Input: part model. Units: mm. Frame: model coordinates. Face numbers are marked on the shaded views. Round coordinates to 2 decimals unless told otherwise and drop trailing zeros. Loops run counter-clockwise (first coordinate to the right, second up) from the corner with the lowest first, then second, coordinate; pieces in that order, holes last. Notation, with made-up numbers: (86.5, -21) - (91.5, -21) arc R29 ccw to (91.5, 17) - close; hole circle Ø8 at (-18, 19). An arc over 180 degrees is marked (long way). One line per question, with ' | ' between items. Start each with the question number.
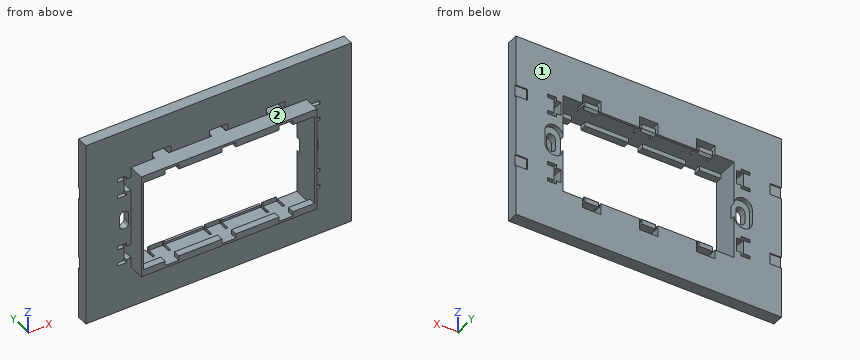
from build123d import *

# Parameters (mm, degrees)
CROQUIS1_W              = 116.45
CROQUIS1_H              = 82
SALIENTE_EXTRUIR2_DEPTH = 5
CROQUIS2_W              = 74.95
CROQUIS2_H              = 44
CORTAR_EXTRUIR1_DEPTH   = 5
CROQUIS3_W              = 76.95
CROQUIS3_H              = 46
CROQUIS3_W_2            = 74.95
CROQUIS3_H_2            = 44
SALIENTE_EXTRUIR3_DEPTH = 7
CROQUIS4_W              = 74.95
CROQUIS4_H              = 3
SALIENTE_EXTRUIR4_DEPTH = 3
CROQUIS5_W              = 3
CROQUIS5_H              = 2
CORTAR_EXTRUIR9_DEPTH   = 3
CROQUIS9_W              = 6
CROQUIS9_H              = 3
CORTAR_EXTRUIR10_DEPTH  = 1
CROQUIS10_W             = 74.95
CROQUIS10_H             = 3
CORTAR_EXTRUIR11_DEPTH  = 1
CROQUIS11_W             = 6
CROQUIS11_H             = 3
CORTAR_EXTRUIR12_DEPTH  = 1
CROQUIS12_W             = 74.95
CROQUIS12_H             = 3
CORTAR_EXTRUIR13_DEPTH  = 1
CROQUIS13_W             = 1
CROQUIS13_H             = 5
CORTAR_EXTRUIR21_DEPTH  = 4
CROQUIS14_W             = 1
CROQUIS14_H             = 5
CORTAR_EXTRUIR22_DEPTH  = 4
CROQUIS15_W             = 8
CROQUIS15_H             = 3
CORTAR_EXTRUIR23_DEPTH  = 16
SALIENTE_EXTRUIR8_DEPTH = 70
SALIENTE_EXTRUIR9_DEPTH = 70
CROQUIS18_W             = 19
CROQUIS18_H             = 42
CORTAR_EXTRUIR24_DEPTH  = 8
CROQUIS19_W             = 9.475
CROQUIS19_H             = 44
CORTAR_EXTRUIR26_DEPTH  = 8
CROQUIS20_W             = 1
CROQUIS20_H             = 44
CORTAR_EXTRUIR27_DEPTH  = 4
CROQUIS21_W             = 5
CROQUIS21_H             = 5
CORTAR_EXTRUIR28_DEPTH  = 0.5
CORTAR_EXTRUIR29_DEPTH  = 5
CORTAR_EXTRUIR30_DEPTH  = 2
CORTAR_EXTRUIR31_DEPTH  = 5


with BuildPart() as part:
    # Croquis1 → Saliente-Extruir2 (new body)
    with BuildSketch(Plane(origin=(0, 0, 0), x_dir=(1, 0, 0), z_dir=(0, 1, 0))):
        Rectangle(CROQUIS1_W, CROQUIS1_H)
    extrude(amount=SALIENTE_EXTRUIR2_DEPTH)

    # Croquis2 → Cortar-Extruir1 (cut)
    with BuildSketch(Plane(origin=(0, 5, 0), x_dir=(1, 0, 0), z_dir=(0, 1, 0))):
        Rectangle(CROQUIS2_W, CROQUIS2_H)
    extrude(amount=-CORTAR_EXTRUIR1_DEPTH, mode=Mode.SUBTRACT)

    # Croquis3 → Saliente-Extruir3 (add)
    with BuildSketch(Plane.XZ):
        Rectangle(CROQUIS3_W, CROQUIS3_H)
        Rectangle(CROQUIS3_W_2, CROQUIS3_H_2, mode=Mode.SUBTRACT)
    extrude(amount=SALIENTE_EXTRUIR3_DEPTH)

    # Croquis4 → Saliente-Extruir4 (add)
    with BuildSketch(Plane.XZ.offset(7)):
        with Locations((0, 20.5)):
            Rectangle(CROQUIS4_W, CROQUIS4_H)
        with Locations((0, -20.5)):
            Rectangle(CROQUIS4_W, CROQUIS4_H)
    extrude(amount=-SALIENTE_EXTRUIR4_DEPTH)

    # Croquis5 → Cortar-Extruir9 (cut)
    with BuildSketch(Plane.XZ.offset(7)):
        Polygon((25, -19), (22, -19), (22, -21), (28, -21), (28, -19), align=None)
        Polygon((22, 21), (22, 19), (25, 19), (28, 19), (28, 21), align=None)
        with Locations((1.5, 20)):
            Rectangle(CROQUIS5_W, CROQUIS5_H)
        with Locations((-1.5, 20)):
            Rectangle(CROQUIS5_W, CROQUIS5_H)
        with Locations((-1.5, -20)):
            Rectangle(CROQUIS5_W, CROQUIS5_H)
        with Locations((1.5, -20)):
            Rectangle(CROQUIS5_W, CROQUIS5_H)
        Polygon((-22, -21), (-22, -19), (-25, -19), (-28, -19), (-28, -21), align=None)
        Polygon((-25, 19), (-22, 19), (-22, 21), (-28, 21), (-28, 19), align=None)
    extrude(amount=-CORTAR_EXTRUIR9_DEPTH, mode=Mode.SUBTRACT)

    # Croquis9 → Cortar-Extruir10 (cut)
    with BuildSketch(Plane(origin=(0, 0, 21), x_dir=(-1, 0, 0), z_dir=(0, 0, -1))):
        with Locations((25, -5.5)):
            Rectangle(CROQUIS9_W, CROQUIS9_H)
        with Locations((0, -5.5)):
            Rectangle(CROQUIS9_W, CROQUIS9_H)
        with Locations((-25, -5.5)):
            Rectangle(CROQUIS9_W, CROQUIS9_H)
    extrude(amount=-CORTAR_EXTRUIR10_DEPTH, mode=Mode.SUBTRACT)

    # Croquis10 → Cortar-Extruir11 (cut)
    with BuildSketch(Plane(origin=(0, 0, 19), x_dir=(-1, 0, 0), z_dir=(0, 0, -1))):
        with Locations((0, -5.5)):
            Rectangle(CROQUIS10_W, CROQUIS10_H)
    extrude(amount=-CORTAR_EXTRUIR11_DEPTH, mode=Mode.SUBTRACT)

    # Croquis11 → Cortar-Extruir12 (cut)
    with BuildSketch(Plane.XY.offset(-21)):
        with Locations((25, -5.5)):
            Rectangle(CROQUIS11_W, CROQUIS11_H)
        with Locations((0, -5.5)):
            Rectangle(CROQUIS11_W, CROQUIS11_H)
        with Locations((-25, -5.5)):
            Rectangle(CROQUIS11_W, CROQUIS11_H)
    extrude(amount=-CORTAR_EXTRUIR12_DEPTH, mode=Mode.SUBTRACT)

    # Croquis12 → Cortar-Extruir13 (cut)
    with BuildSketch(Plane.XY.offset(-19)):
        with Locations((0, -5.5)):
            Rectangle(CROQUIS12_W, CROQUIS12_H)
    extrude(amount=-CORTAR_EXTRUIR13_DEPTH, mode=Mode.SUBTRACT)

    # Croquis13 → Cortar-Extruir21 (cut)
    with BuildSketch(Plane.XY.offset(-22)):
        with Locations((21.5, 2.5)):
            Rectangle(CROQUIS13_W, CROQUIS13_H)
        with Locations((3.5, 2.5)):
            Rectangle(CROQUIS13_W, CROQUIS13_H)
        with Locations((-3.5, 2.5)):
            Rectangle(CROQUIS13_W, CROQUIS13_H)
        with Locations((-28.5, 2.5)):
            Rectangle(CROQUIS13_W, CROQUIS13_H)
        with Locations((-21.5, 2.5)):
            Rectangle(CROQUIS13_W, CROQUIS13_H)
        with Locations((28.5, 2.5)):
            Rectangle(CROQUIS13_W, CROQUIS13_H)
    extrude(amount=-CORTAR_EXTRUIR21_DEPTH, mode=Mode.SUBTRACT)

    # Croquis14 → Cortar-Extruir22 (cut)
    with BuildSketch(Plane(origin=(0, 0, 22), x_dir=(-1, 0, 0), z_dir=(0, 0, -1))):
        with Locations((28.5, 2.5)):
            Rectangle(CROQUIS14_W, CROQUIS14_H)
        with Locations((-21.5, 2.5)):
            Rectangle(CROQUIS14_W, CROQUIS14_H)
        with Locations((21.5, 2.5)):
            Rectangle(CROQUIS14_W, CROQUIS14_H)
        with Locations((3.5, 2.5)):
            Rectangle(CROQUIS14_W, CROQUIS14_H)
        with Locations((-3.5, 2.5)):
            Rectangle(CROQUIS14_W, CROQUIS14_H)
        with Locations((-28.5, 2.5)):
            Rectangle(CROQUIS14_W, CROQUIS14_H)
    extrude(amount=-CORTAR_EXTRUIR22_DEPTH, mode=Mode.SUBTRACT)

    # Croquis15 → Cortar-Extruir23 (cut)
    with BuildSketch(Plane.XZ):
        with Locations((0, 24.5)):
            Rectangle(CROQUIS15_W, CROQUIS15_H)
        with Locations((-25, 24.5)):
            Rectangle(CROQUIS15_W, CROQUIS15_H)
        with Locations((25, 24.5)):
            Rectangle(CROQUIS15_W, CROQUIS15_H)
        with Locations((-25, -24.5)):
            Rectangle(CROQUIS15_W, CROQUIS15_H)
        with Locations((0, -24.5)):
            Rectangle(CROQUIS15_W, CROQUIS15_H)
        with Locations((25, -24.5)):
            Rectangle(CROQUIS15_W, CROQUIS15_H)
    extrude(amount=-CORTAR_EXTRUIR23_DEPTH, mode=Mode.SUBTRACT)

    # Croquis16 → Saliente-Extruir8 (add)
    with BuildSketch(Plane.ZY.offset(-37.475)):
        Polygon((-22, 5), (-21, 5), (-20, 4), (-22, 4), align=None)
    extrude(amount=SALIENTE_EXTRUIR8_DEPTH)

    # Croquis17 → Saliente-Extruir9 (add)
    with BuildSketch(Plane.ZY.offset(-37.475)):
        Polygon((22, 4), (22, 5), (21, 5), (20, 4), (21, 4), align=None)
    extrude(amount=SALIENTE_EXTRUIR9_DEPTH)

    # Croquis18 → Cortar-Extruir24 (cut)
    with BuildSketch(Plane(origin=(0, 5, 0), x_dir=(1, 0, 0), z_dir=(0, 1, 0))):
        with Locations((-12.5, 0)):
            Rectangle(CROQUIS18_W, CROQUIS18_H)
        with Locations((12.5, 0)):
            Rectangle(CROQUIS18_W, CROQUIS18_H)
    extrude(amount=-CORTAR_EXTRUIR24_DEPTH, mode=Mode.SUBTRACT)

    # Croquis19 → Cortar-Extruir26 (cut)
    with BuildSketch(Plane(origin=(0, 5, 0), x_dir=(1, 0, 0), z_dir=(0, 1, 0))):
        with Locations((32.7375, 0)):
            Rectangle(CROQUIS19_W, CROQUIS19_H)
        with Locations((-32.7375, 0)):
            Rectangle(CROQUIS19_W, CROQUIS19_H)
    extrude(amount=-CORTAR_EXTRUIR26_DEPTH, mode=Mode.SUBTRACT)

    # Croquis20 → Cortar-Extruir27 (cut)
    with BuildSketch(Plane(origin=(0, 5, 0), x_dir=(1, 0, 0), z_dir=(0, 1, 0))):
        with Locations((-3.5, 0)):
            Rectangle(CROQUIS20_W, CROQUIS20_H)
        with Locations((-21.5, 0)):
            Rectangle(CROQUIS20_W, CROQUIS20_H)
        with Locations((3.5, 0)):
            Rectangle(CROQUIS20_W, CROQUIS20_H)
        with Locations((21.5, 0)):
            Rectangle(CROQUIS20_W, CROQUIS20_H)
    extrude(amount=-CORTAR_EXTRUIR27_DEPTH, mode=Mode.SUBTRACT)

    # Croquis21 → Cortar-Extruir28 (cut)
    with BuildSketch(Plane(origin=(0, 5, 0), x_dir=(1, 0, 0), z_dir=(0, 1, 0))):
        Polygon((-53.225, -13.5), (-58.225, -13.5), (-58.225, -18.5), (-53.225, -18.5), (-53.225, -16), align=None)
        Polygon((-53.225, 18.5), (-58.225, 18.5), (-58.225, 13.5), (-53.225, 13.5), (-53.225, 16), align=None)
        Polygon((53.225, -18.5), (58.225, -18.5), (58.225, -13.5), (53.225, -13.5), (53.225, -16), align=None)
        with Locations((55.725, 16)):
            Rectangle(CROQUIS21_W, CROQUIS21_H)
    extrude(amount=-CORTAR_EXTRUIR28_DEPTH, mode=Mode.SUBTRACT)

    # Croquis22 → Cortar-Extruir29 (cut)
    with BuildSketch(Plane(origin=(0, 5, 0), x_dir=(1, 0, 0), z_dir=(0, 1, 0))):
        with BuildLine():
            Line((-39.475, -2), (-39.475, 2))
            ThreePointArc((-39.475, 2), (-41.475, 4), (-43.475, 2))
            Line((-43.475, 2), (-43.475, -2))
            ThreePointArc((-43.475, -2), (-41.475, -4), (-39.475, -2))
        make_face()
        with BuildLine():
            ThreePointArc((43.475, -2), (41.475, -4), (39.475, -2))
            Line((39.475, -2), (39.475, 2))
            ThreePointArc((39.475, 2), (41.475, 4), (43.475, 2))
            Line((43.475, 2), (43.475, -2))
        make_face()
    extrude(amount=-CORTAR_EXTRUIR29_DEPTH, mode=Mode.SUBTRACT)

    # Croquis23 → Cortar-Extruir30 (cut)
    with BuildSketch(Plane(origin=(0, 5, 0), x_dir=(1, 0, 0), z_dir=(0, 1, 0))):
        with BuildLine():
            Line((-37.475, 0), (-37.475, 3))
            ThreePointArc((-37.475, 3), (-41.475, 7), (-45.475, 3))
            Line((-45.475, 3), (-45.475, -3))
            ThreePointArc((-45.475, -3), (-41.475, -7), (-37.475, -3))
            Line((-37.475, -3), (-37.475, 0))
        make_face()
        with BuildLine():
            ThreePointArc((45.475, -3), (41.475, -7), (37.475, -3))
            Line((37.475, -3), (37.475, 0))
            Line((37.475, 0), (37.475, 3))
            ThreePointArc((37.475, 3), (41.475, 7), (45.475, 3))
            Line((45.475, 3), (45.475, -3))
        make_face()
    extrude(amount=-CORTAR_EXTRUIR30_DEPTH, mode=Mode.SUBTRACT)

    # Croquis24 → Cortar-Extruir31 (cut)
    with BuildSketch(Plane(origin=(0, 5, 0), x_dir=(1, 0, 0), z_dir=(0, 1, 0))):
        Polygon((-38.475, -12.5), (-38.475, -18.5), (-40.475, -18.5), (-40.475, -20), (-44.475, -20), (-44.475, -18.5), (-41.475, -18.5), (-41.475, -12.5), (-44.475, -12.5), (-44.475, -11), (-40.475, -11), (-40.475, -12.5), align=None)
        Polygon((-38.475, 12.5), (-40.475, 12.5), (-40.475, 11), (-44.475, 11), (-44.475, 12.5), (-41.475, 12.5), (-41.475, 18.5), (-44.475, 18.5), (-44.475, 20), (-40.475, 20), (-40.475, 18.5), (-38.475, 18.5), align=None)
        Polygon((38.475, 12.5), (38.475, 18.5), (40.475, 18.5), (40.475, 20), (44.475, 20), (44.475, 18.5), (41.475, 18.5), (41.475, 12.5), (44.475, 12.5), (44.475, 11), (40.475, 11), (40.475, 12.5), align=None)
        Polygon((38.475, -12.5), (40.475, -12.5), (40.475, -11), (44.475, -11), (44.475, -12.5), (41.475, -12.5), (41.475, -18.5), (44.475, -18.5), (44.475, -20), (40.475, -20), (40.475, -18.5), (38.475, -18.5), align=None)
    extrude(amount=-CORTAR_EXTRUIR31_DEPTH, mode=Mode.SUBTRACT)


solid = part.part
(1) Section B-B, the plane z = -34. Output: boundary loops of the cut face in (x, y) (3 decimals).
(2) Line query: line 1 along X through (y, z) = (2, 16.5) (3 decimals); line 2 along X through (y, z) = (4.5, 25) (3 decimals); line 3 along X through (y, z) = (-4.25, 9.5) (3 decimals). Output: solid intervals per line, ascending. Write a range as from..to.
(3) Pull-direction query (Z, two-part tool) for the marked faces 1 and 2; classes: released by +Z, released by -Z, zero draft, split by the parting line, or undercut.
(4) Section A-A, the plane z = -16. Output: boundary loops of the cut face in (x, y) (3 decimals).
(5) Pin query (flat end, axial travel): P1, Ø2, axis at y = -5, z = 21, coming from the +X side (3 decimals); P2, Ø0.6, axis at y = -5, z = 21, coming from the -X side (3 decimals). Return the tip coordinate at first contact, or that it passes through.
Derived:
1) outline: (-58.225, 0) - (58.225, 0) - (58.225, 5) - (-58.225, 5) - close
2) line 1: x = -58.225..-41.475, -38.475..-37.475, 37.475..38.475, 41.475..58.225 | line 2: x = -58.225..-29, -21..-4, 4..21, 29..58.225 | line 3: x = -38.475..-37.475, 37.475..38.475
3) face 1: zero draft | face 2: undercut
4) outline: (-58.225, 0) - (-41.475, 0) - (-41.475, 5) - (-53.225, 5) - (-53.225, 4.5) - (-58.225, 4.5) - close; (-38.475, -7) - (-37.475, -7) - (-37.475, 5) - (-38.475, 5) - close; (37.475, -7) - (38.475, -7) - (38.475, 5) - (37.475, 5) - close; (41.475, 0) - (58.225, 0) - (58.225, 4.5) - (53.225, 4.5) - (53.225, 5) - (41.475, 5) - close
5) P1: stops at x = 38.475 | P2: stops at x = -38.475
